Input: part model. Units: mm. Frame: model coordinates. Round coordinates to 2 decimals unless told otherwise and drop trailing zeros. Loops run counter-clockwise (first coordinate to the right, second up) from the corner with the lowest first, then second, coordinate; pieces in that order, holes last.
(1) Cut plane A-A, the plane x = 28.5. Output: boundary loops of the cut face in (y, z), and give its area (3 significant figures).
(2) Cut plane B-B, the plane z = 0.25. Output: boundary loops of the cut face in (x, y), and give its area (3 significant figures).
(3) Line query: line 1 (Y direction, x = -15.5, z = 0.55). Output: solid intervals per line, ascending.
(4) Cut plane C-C, the plane y = 0. Give the number of separate pieces and of enclosed holes in the cut face, and give its area (3 significant figures).
from build123d import *

# Parameters (mm, degrees)
F0_R     = 1.5
F0_W     = 13
F0_H     = 3
F1_DEPTH = 1


with BuildPart() as f1:
    # F0 (on Top) → F1 (new body)
    with BuildSketch(Plane.XY):
        Polygon((0, 1.5), (0, 3), (-55, 3), (-55, 1.5), (-31.5, 1.5), (-31.5, -1.5), (-55, -1.5), (-55, -3), (0, -3), (0, -1.5), (-6.5, -1.5), (-6.5, 1.5), align=None)
        with Locations((-28.5, 0)):
            Circle(F0_R, mode=Mode.SUBTRACT)
        with Locations((-19, 0)):
            Rectangle(F0_W, F0_H, mode=Mode.SUBTRACT)
        with Locations((-9.5, 0)):
            Circle(F0_R, mode=Mode.SUBTRACT)
        Polygon((55, 3), (0, 3), (0, 1.5), (6.5, 1.5), (6.5, -1.5), (0, -1.5), (0, -3), (55, -3), (55, -1.5), (31.5, -1.5), (31.5, 1.5), (55, 1.5), align=None)
        with Locations((9.5, 0)):
            Circle(F0_R, mode=Mode.SUBTRACT)
        with Locations((19, 0)):
            Rectangle(F0_W, F0_H, mode=Mode.SUBTRACT)
        with Locations((28.5, 0)):
            Circle(F0_R, mode=Mode.SUBTRACT)
    extrude(amount=F1_DEPTH)


solid = f1.part
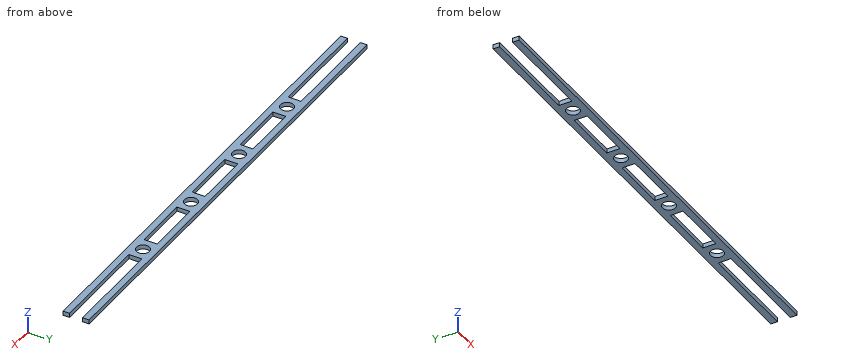
Reported:
1. outline: (-3, 0) - (-1.5, 0) - (-1.5, 1) - (-3, 1) - close; (1.5, 0) - (3, 0) - (3, 1) - (1.5, 1) - close
1. area: 3.00 mm2
2. outline: (-55, -3) - (55, -3) - (55, -1.5) - (31.5, -1.5) - (31.5, 1.5) - (55, 1.5) - (55, 3) - (-55, 3) - (-55, 1.5) - (-31.5, 1.5) - (-31.5, -1.5) - (-55, -1.5) - close; hole circle Ø3 at (-28.5, 0); hole (-25.5, -1.5) - (-12.5, -1.5) - (-12.5, 1.5) - (-25.5, 1.5) - close; hole circle Ø3 at (-9.5, 0); hole (-6.5, -1.5) - (6.5, -1.5) - (6.5, 1.5) - (-6.5, 1.5) - close; hole circle Ø3 at (9.5, 0); hole (12.5, -1.5) - (25.5, -1.5) - (25.5, 1.5) - (12.5, 1.5) - close; hole circle Ø3 at (28.5, 0)
2. area: 374 mm2
3. line 1: y = -3 to -1.5, 1.5 to 3
4. separate pieces: 8
4. enclosed holes: 0
4. area: 12.0 mm2
